Source: CAD feature listing. Evaluate the final solid. Frame: model axes, mm. Give positions to 0.01 mm unless a question says otherwise; leave off trailing zeros. Write each loop counter-clockwise with the first axis right and the second up, starting at its lowest first coordinate (ties: lowest second). Pieces come first, ordered by that corner, then holes. Notation, with made-up numbers: (81.25, -39.5) -> (135.25, -39.5) arc R23 ccw to (135.25, -27.5) -> close; hole circle Ø8 at (68.25, 87). An arc over 180 degrees is marked (long way). Use one line per item in the form item = value. Start each with the question number.
(1) Material intervals for line 1 along Y through (x, z) = (-27, 1.35); line 2 along X through (y, z) = (47, 3.5); line 3 along Y through (x, z) = (-23, 3.85), sorted ascending. Write a range as from..to.
(2) Cut plane A-A, the plane x = -26.5. Output: boundary loops of the cut face in (y, z).
(3) First-contact query: P1, Ø8, axis at x = -16, y = 37.5, coming from the -Z side. Flat tip, straight axial feed; report the tip coordinate or a pass-through.
from build123d import *

# Parameters (mm, degrees)
ESQUISSE1_W      = 25
ESQUISSE1_H      = 80
EXTRUSION1_DEPTH = 6
CONG_1_R         = 10


with BuildPart() as part:
    # Esquisse1 → Extrusion1 (new body)
    with BuildSketch(Plane.XY):
        with Locations((-17.5, 10)):
            Rectangle(ESQUISSE1_W, ESQUISSE1_H)
    extrude(amount=EXTRUSION1_DEPTH)

    # Congé1
    cong_1_edges = [part.edges().sort_by_distance(p)[0] for p in [
        (-30, 50, 3),
    ]]
    fillet(cong_1_edges, radius=CONG_1_R)


solid = part.part
Geometry says:
q1.line_1 = -30..47.14
q1.line_2 = -27.14..-5
q1.line_3 = -30..49.54
q2.outline = (-30, 0) -> (47.6, 0) -> (47.6, 6) -> (-30, 6) -> close
q3.P1 = 0
